Design review of the part shown in the three views and the two pictorial views. Dimensions are in mm from the part's minimum x, y and z. Round coordinates to 2 decimals unless told otherwise and drop trailing zeros. Order: outer loops, then holes, each group sorted by start corner. A loop starts at its lowest first (then second) coordinate and runs counter-clockwise, first axis right, second up. Notation, with made-up numbers: M 62,61.5 L 95,61.5 A13 ccw 95,71.5 Z; hole C 36.25,86 d7. An arc over 180 degrees is marked long. Use a Markdown table: item, result. Add a question column.
(1) Take a section at C-C (x = 7.25). Write out the cut boundary in (y, z) (1 decimal), then the cut area to 3 significant figures.
(2) Take a section at A-A (z = 27.5). Write out the cut boundary in (x, y) (1 decimal), then the cut area to 3 significant figures.
(3) For pin 1 (5 mm diameter, centred on x = 7, y = 20.5, fed in from +Z); pin 2 (1.5 mm diameter, centred on x = 10.5, z = 189, fed in from +Y); pin 3 (2 mm diameter, centred on x = 3, z = 112, fed in from -Y); pin 4 (11.5 mm diameter, centred on y = 15, z = 27.5, fed in from -X), all flat-tipped, find the tip position at first contact; note any pin that passes through.
(4) To check wall thickness, follow probe 1 along Z at (x, y) = (10.75, 15); probe 2 along Z at (x, y) = (7.75, 60); probe 3 along Z at (x, y) = (5, 112). State the ranges of each line that lie inside material, in increasing order. Write a range as from..to.
(5) Take a section at B-B (y = 60). Write out the cut boundary in (x, z) (1 decimal), then the cut area to 4 significant figures.
(6) Take a section at D-D (y = 15). Write out the cut boundary in (x, z) (1 decimal).
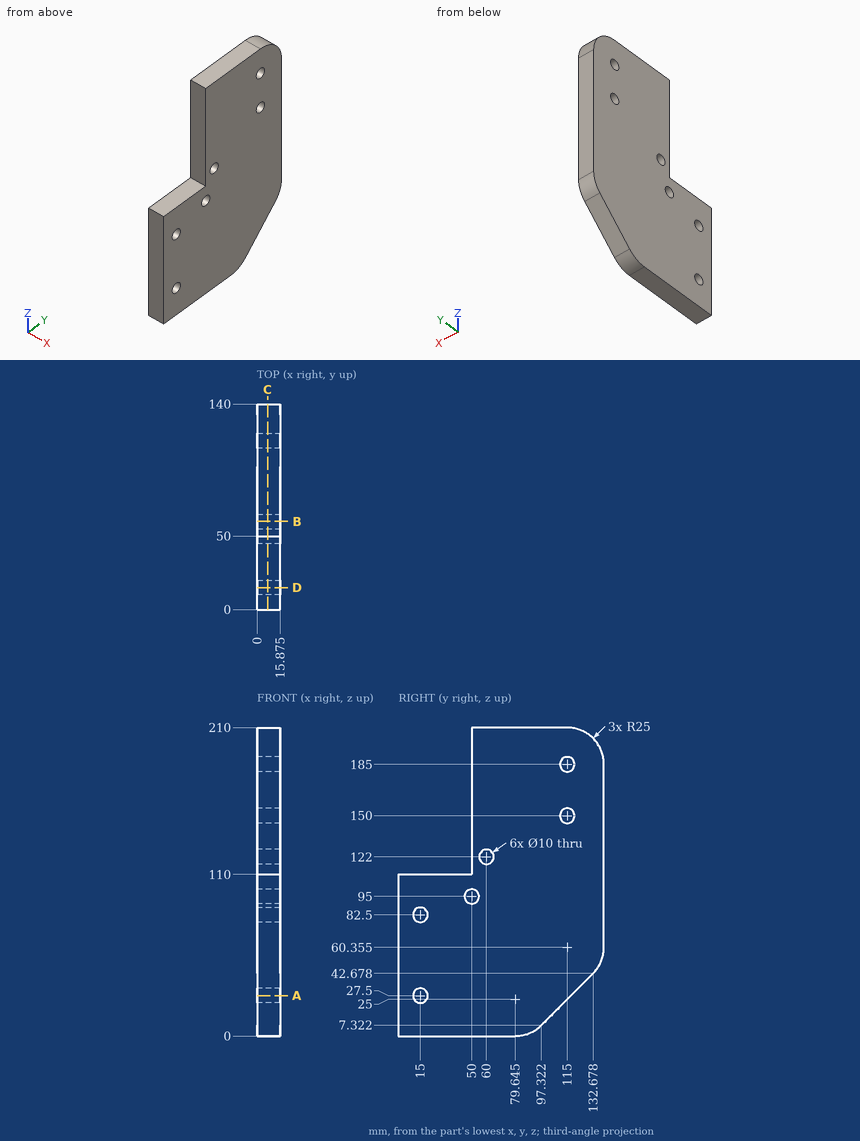
Verdict:
| question | item | result |
|---|---|---|
| 1 | outline | M 0,0 L 79.6,0 A25 ccw 97.3,7.3 L 132.7,42.7 A25 ccw 140,60.4 L 140,185 A25 ccw 115,210 L 50,210 L 50,110 L 0,110 Z; hole C 15,27.5 d10; hole C 15,82.5 d10; hole C 50,95 d10; hole C 60,122 d10; hole C 115,150 d10; hole C 115,185 d10 |
| 1 | area | 22,500 mm^2 |
| 2 | outline | M 0,0 L 15.9,0 L 15.9,10 L 0,10 Z; M 0,20 L 15.9,20 L 15.9,117.5 L 0,117.5 Z |
| 2 | area | 1,710 mm^2 |
| 3 | pin 1 | stops at z = 110 |
| 3 | pin 2 | stops at y = 139.79 |
| 3 | pin 3 | stops at y = 50 |
| 3 | pin 4 | stops at x = 0 |
| 4 | probe 1 | z = 0..22.5, 32.5..77.5, 87.5..110 |
| 4 | probe 2 | z = 0..117, 127..210 |
| 4 | probe 3 | z = 22..146, 154..181, 189..210 |
| 5 | outline | M 0,0 L 15.9,0 L 15.9,117 L 0,117 Z; M 0,127 L 15.9,127 L 15.9,210 L 0,210 Z |
| 5 | area | 3,175 mm^2 |
| 6 | outline | M 0,0 L 15.9,0 L 15.9,22.5 L 0,22.5 Z; M 0,32.5 L 15.9,32.5 L 15.9,77.5 L 0,77.5 Z; M 0,87.5 L 15.9,87.5 L 15.9,110 L 0,110 Z |
